Check sheet for the modelled part. Datum: model origin and axes. Units: mm. A direction names the side the tool comes from. Give positions to 0.01 mm unless a question says otherwise; leave off trailing zeros. Order: outer loops, then holes, each group sorted by start corner. A loop starts at its lowest first (then second) coordinate and runs counter-clockwise, first axis right, second up.
Autodesk Fusion 360 part; units mm, degrees
sketch "Sketch1" plane through (0, 0, 0) normal (1, 0, 0) x (0, 1, 0)
  circle A0 centre (0, 0) radius 20
  line L0 (0, 0) -> (65, -112.5833)
  line L1 (0, 0) -> (130, 0) construction
  line L2 (-16.4974, -11.3065) -> (56.3397, -117.5833)
  line L3 (56.3397, -117.5833) -> (65, -112.5833)
  line L4 (65, -112.5833) -> (73.6603, -107.5833)
  line L5 (73.6603, -107.5833) -> (18.0404, 8.6339)
  circle A1 centre (0, 0) radius 17.5
  circle A2 centre (61.25, -106.0881) radius 12.5
  circle A3 centre (61.25, -106.0881) radius 7.5
  dimension "d1" = 40
  dimension "d2" = 60
  dimension "d3" = 130
  dimension "d4" = 10
  dimension "d5" = 10
  dimension "d6" = 35
  dimension "d7" = 25
  dimension "d8" = 15
extrude "Extrude1" add sketch "Sketch1" along normal mid plane 8 contours A1 | A0 | A0 L0 L5 A2 | A0 L0 L2 A2 | L0 L4 L5 A2 A3 | L0 L2 L3 A2 A3 | L3 L4 A2 | L0 A3 | L0 A3
extrude "Extrude2" add sketch "Sketch1" against normal blind 15 contours A1
extrude "Extrude3" add sketch "Sketch1" along normal mid plane 20 contours L0 A3 | L0 A3
extrude "Extrude4" cut 1 faces at (10, 60.7061, -108.3596) along direction (-1, 0, 0) blind 6
extrude "Extrude5" cut 1 faces at (-10, 60.6937, -103.8711) along direction (1, 0, 0) blind 6
sketch "Sketch2" plane through (-15, 0, 0) normal (-1, 0, 0) x (0, -1, 0)
  circle A0 centre (0, 0) radius 17.5
  line L0 (0, 0) -> (0, 10.5)
  line L1 (0, 0) -> (0, -10.5)
  circle A1 centre (0, 10.5) radius 1
  circle A2 centre (0, -10.5) radius 1
  dimension "d19" = 10.5
  dimension "d20" = 10.5
  dimension "d21" = 2
  dimension "d22" = 2
extrude "Extrude6" cut sketch "Sketch2" against normal blind 26 contours A1 | A2
sketch "Sketch3" plane through (-15, 0, 0) normal (-1, 0, 0) x (0, -1, 0)
  circle A0 centre (0, 10.5) radius 1
  circle A1 centre (0, -10.5) radius 1
  circle A2 centre (0, 0) radius 17.5
  circle A3 centre (0, 0) radius 15.5
  dimension "d25" = 31
extrude "Extrude7" cut sketch "Sketch3" against normal blind 2 contours A3
sketch "Sketch4" plane through (4, 0, 0) normal (1, 0, 0) x (0, 1, 0)
  circle A0 centre (0, 10.5) radius 1
  circle A1 centre (0, -10.5) radius 1
  line L0 (73.6603, -107.5833) -> (18.0404, 8.6339)
  arc A2 (18.0404, 8.6339) -> (-16.4974, -11.3065) centre (0, 0) ccw
  line L1 (-16.4974, -11.3065) -> (56.3397, -117.5833)
  arc A3 (56.3397, -117.5833) -> (73.6603, -107.5833) centre (61.25, -106.0881) ccw
  circle A4 centre (0, 0) radius 15.5
  circle A5 centre (0, 0) radius 15.5
extrude "Extrude8" cut sketch "Sketch4" against normal blind 10 contours A4 A5
sketch "Sketch5" plane through (4, 0, 0) normal (1, 0, 0) x (0, 1, 0)
  circle A0 centre (0, 0) radius 15.5
  line L0 (73.6603, -107.5833) -> (18.0404, 8.6339)
  arc A1 (18.0404, 8.6339) -> (-16.4974, -11.3065) centre (0, 0) ccw
  line L1 (-16.4974, -11.3065) -> (56.3397, -117.5833)
  arc A2 (56.3397, -117.5833) -> (73.6603, -107.5833) centre (61.25, -106.0881) ccw
  circle A3 centre (61.25, -106.0881) radius 12.5
  circle A4 centre (61.25, -106.0881) radius 4
  dimension "d30" = 8
extrude "Extrude9" cut sketch "Sketch5" against normal blind 10 contours A4
equation "d19 = ( 21 / 2 ) * 1 mm"
(1) Cross-section at C-C on z = -1.5. Enter the section's corners in (x, y).
Response values:
outline: (-15, -17.44) - (-4, -17.44) - (-4, -19.94) - (4, -19.94) - (4, -15.43) - (-6, -15.43) - (-6, 15.43) - (4, 15.43) - (4, 22.89) - (-4, 22.89) - (-4, 17.44) - (-15, 17.44) - (-15, 15.43) - (-13, 15.43) - (-13, -15.43) - (-15, -15.43) - close
(2) Material ranges on L1, parallel to Z at x = -10, y = 0; L2, parallel to X at y = 55.5, z = -112; L3, parallel to Y at x = -1, z = -108, recorded low to high.
Response values:
L1: z = -17.5 to -11.5, -9.5 to 9.5, 11.5 to 17.5
L2: x = -4 to 4
L3: y = 49.77 to 57.74, 64.76 to 73.6
(3) Release check for a two-part mould opening along Y. For faces 1 (the face through (0.056, 64.945, -107.62)), 2 (the face through (4, 30, -49)), 3 (the face through (-0.06, 46.24, -50.29)) record: released by +Y, released by -Y, zero draft, split by the parting line, or undercut.
Response values:
face 1: undercut
face 2: zero draft
face 3: released by +Y
(4) Set-up check for faces 4 (the face through (-6, 0, 0)), 5 (the face through (-13, 0, 0)), 6 (the face through (-0.06, 19.41, -63.7)): record each of +Z, -Z, +X, -X, +Y, -Y from which the full face is reachable in a straight line by a thin tool's end or side.
Response values:
face 4: +X
face 5: -X
face 6: -Z, +X, -X, -Y
(5) Gauge pin test, flat ends, axial feed: pin 1 Ø9.5 at (y, z) = (5, 7.5) entering from +X; pin 2 Ø2 at (x, z) = (2, -97) entering from +Y; pin 3 Ø2.5 at (y, z) = (0, 10.5) entering from -X. Record the tip position at first contact, or that the pin passes through.
Response values:
pin 1: stops at x = -6
pin 2: stops at y = 69.07
pin 3: stops at x = -13
(6) Cross-section at B-B on x = 1. Enter the section's corners in (y, z).
Response values:
outline: (-16.5, -11.31) - (56.34, -117.58) arc R12.5 ccw to (73.66, -107.58) - (18.04, 8.63) arc R20 ccw (long way) to start; hole circle Ø31 at (0, 0); hole circle Ø8 at (61.25, -106.09)
(7) Cross-section at A-A on y = 61.25. Enter the section's corners in (x, z).
Response values:
outline: (-4, -118.59) - (4, -118.59) - (4, -110.09) - (-4, -110.09) - close; (-4, -102.09) - (4, -102.09) - (4, -81.65) - (-4, -81.65) - close
(8) Cross-section at D-D on y = -5.5. Enter the section's corners in (x, z).
Response values:
outline: (-15, -16.61) - (-4, -16.61) - (-4, -27.35) - (4, -27.35) - (4, -14.49) - (-6, -14.49) - (-6, 14.49) - (4, 14.49) - (4, 19.23) - (-4, 19.23) - (-4, 16.61) - (-15, 16.61) - (-15, 14.49) - (-13, 14.49) - (-13, -14.49) - (-15, -14.49) - close
